```python
from build123d import *

# Parameters (mm, degrees)
BOSS_EXTRUDE1_DEPTH = 125
SKETCH3_W           = 257.3
SKETCH3_H           = 237.3
CUT_EXTRUDE1_DEPTH  = 1000
BOSS_EXTRUDE2_DEPTH = 135
SHELL1_START        = -125
SHELL1_DEPTH        = 250
SKETCH6_R           = 6.5
CUT_EXTRUDE2_DEPTH  = 30


# Read off the part's stored shape, not the designer's step: Shell1
with BuildPart() as part:
    # Sketch2 → Boss-Extrude1 (new, symmetric)
    with BuildSketch(Plane.XY):
        Polygon((-135, 0), (135, 0), (185, 0), (185, 6.35), (135, 6.35), (135, 845), (-135, 845), (-135, 6.35), (-185, 6.35), (-185, 0), align=None)
    extrude(amount=BOSS_EXTRUDE1_DEPTH, both=True)

    # Sketch3 → Cut-Extrude1 (cut)
    with BuildSketch(Plane(origin=(0, 845, 0), x_dir=(1, 0, 0), z_dir=(0, 1, 0))):
        Rectangle(SKETCH3_W, SKETCH3_H)
    extrude(amount=-CUT_EXTRUDE1_DEPTH, mode=Mode.SUBTRACT)

    # Sketch5 → Boss-Extrude2 (add, symmetric)
    with BuildSketch(Plane(origin=(0, 0, 0), x_dir=(0, 0, -1), z_dir=(1, 0, 0))):
        Polygon((-125, 865), (325.311522824, 1180.311522824), (325.311522824, 1045.311522824), (125, 845), (-125, 845), align=None)
    extrude(amount=BOSS_EXTRUDE2_DEPTH, both=True)

    # Shell1 outline → Shell1 (cut)
    with BuildSketch(Plane.YZ.offset(SHELL1_START)):
        Polygon((855, 115), (855, -120.857864376), (1059.453658448, -325.311522824), (1168.103776937, -325.311522824), (859.794329494, 115), align=None)
    extrude(amount=SHELL1_DEPTH, mode=Mode.SUBTRACT)

    # Sketch6 → Cut-Extrude2 (cut)
    with BuildSketch(Plane.XZ):
        with Locations((150, 75)):
            Circle(SKETCH6_R)
        with Locations(Location((150, -75, 0), (0, 0, 270))):
            Circle(SKETCH6_R)
        with Locations((-150, 75)):
            Circle(SKETCH6_R)
        with Locations((-150, -75)):
            Circle(SKETCH6_R)
    extrude(amount=-CUT_EXTRUDE2_DEPTH, mode=Mode.SUBTRACT)


solid = part.part
```
Here's how the part is built. I have some questions about the finished solid (model axes, mm). A direction names the side the tool comes from. Coordinates: 2 decimals unless noted, no trailing zeros. Order: outer loops, then holes, each group sorted by start corner. A loop starts at its lowest first (then second) coordinate and runs counter-clockwise, first axis right, second up.
1) We'd pull the mould along Y, two halves only. Please class faces 1 (the face through (125, 975, -151)), 2 (the face through (2, 845, -2)), 3 (the face through (160, 6.35, 2)): +Y half, -Y half, draft (parallel to the pull), parting line (faces both ways), or undercut.
2) Will these pins go through, and if not, where does the flat tip stop? pin 1 (2.5 mm diameter, centred on x = -58, y = 857.5, fed in from -Z); pin 2 (1 mm diameter, centred on x = -30, y = 623.5, fed in from -Z); pin 3 (15 mm diameter, centred on x = -150, z = -75, fed in from +Y); pin 4 (10.5 mm diameter, centred on x = 150, z = 75, fed in from +Y).
3) Which directions (+Z, -Z, +X, -X, +Y, -Y) give clear straight access to the entire face, cutting with the end or side of a thin tool? Please do faces 4 (the face through (-3, 428, -125)), 5 (the face through (-125, 975, -151)), 6 (the face through (-160, 6.35, 2)), 7 (the face through (-128.65, 428, 2)).
4) Imagine slicing it at C-C on x = 23. List the corners of the cut face in (y, z) for me, and give its area (3 significant figures).
5) Imagine slicing it at A-A on y = 691. List the corners of the cut face in (x, z) for me, and give its area (3 significant figures).
6) Imagine slicing it at D-D on y = 1085.5. List the corners of the cut face in (x, z) for me.
7) Imagine slicing it at B-B on z = -193. List the corners of the cut face in (x, y) for me, and give its area (3 significant figures).
8) I need wall thicknesses on line 1 (Z direction, x = -150, y = 4); line 2 (Z direction, x = -64, y = 382); line 3 (X direction, y = 308, z = -81). Which ranges of each line are inside material? Lowest first, please.
Response values:
1. face 1: undercut
1. face 2: -Y half
1. face 3: +Y half
2. pin 1: stops at z = -138.75
2. pin 2: stops at z = -125
2. pin 3: stops at y = 6.35
2. pin 4: passes through
3. face 4: -Z, +X, -X, -Y
3. face 5: none
3. face 6: +Z, -Z, -X, +Y
3. face 7: -Y
4. outline: (0, -125) - (845, -125) - (1045.31, -325.31) - (1059.45, -325.31) - (855, -120.86) - (855, 115) - (859.79, 115) - (1168.1, -325.31) - (1180.31, -325.31) - (865, 125) - (0, 125) - (0, 118.65) - (845, 118.65) - (845, -118.65) - (0, -118.65) - close
4. area: 21,600 mm2
5. outline: (-135, -125) - (135, -125) - (135, 125) - (-135, 125) - close; hole (-128.65, -118.65) - (128.65, -118.65) - (128.65, 118.65) - (-128.65, 118.65) - close
5. area: 6,440 mm2
6. outline: (-135, -325.31) - (-125, -325.31) - (-125, -207.34) - (125, -207.34) - (125, -325.31) - (135, -325.31) - (135, -189.91) - (-135, -189.91) - close
7. outline: (-135, 913) - (135, 913) - (135, 1087.67) - (-135, 1087.67) - close; hole (-125, 927.14) - (125, 927.14) - (125, 1075.46) - (-125, 1075.46) - close
7. area: 10,100 mm2
8. line 1: z = -125 to -81.5, -68.5 to 68.5, 81.5 to 125
8. line 2: z = -125 to -118.65, 118.65 to 125
8. line 3: x = -135 to -128.65, 128.65 to 135
